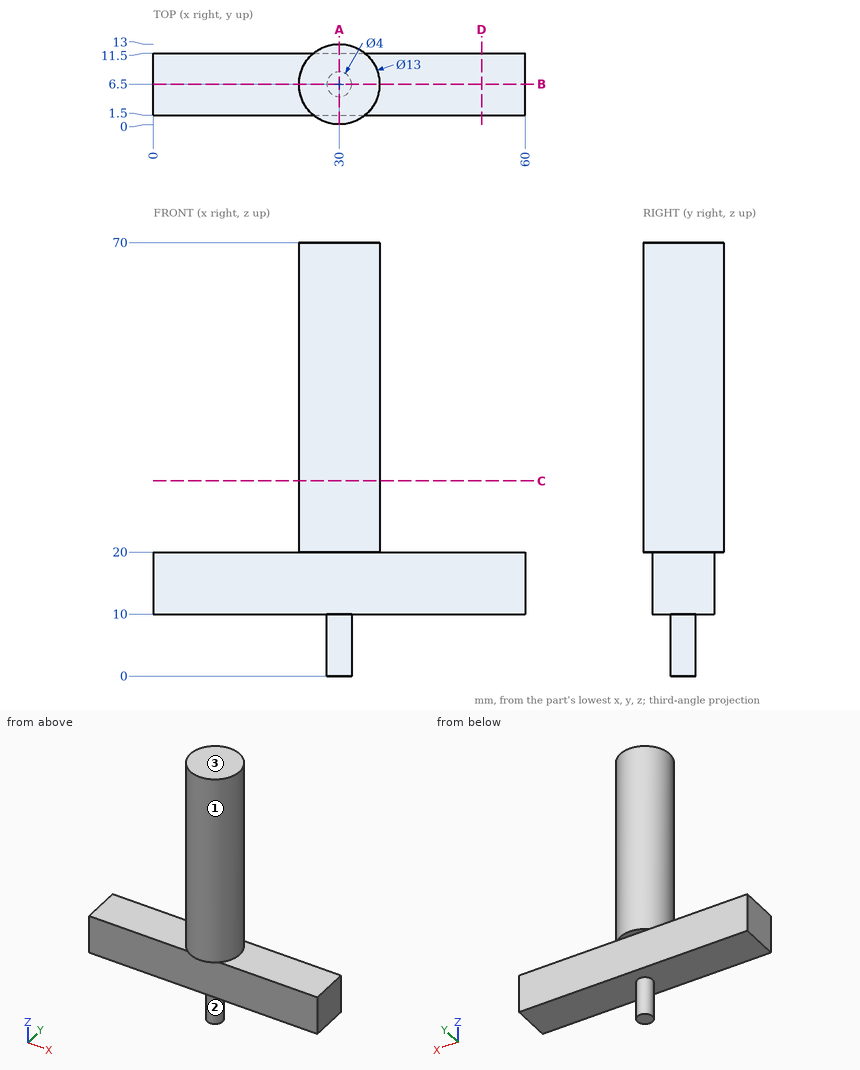
Geometry: see drawing. Coordinates: mm, zero at the bounding-box minimum. A direction names the side the tool comes from. Round coordinates to 2 decimals unless told otherwise and drop trailing zeros. Loops run counter-clockwise (first coordinate to the right, second up) from the corner with the lowest first, then second, coordinate; pieces in that order, holes last. Notation, with made-up numbers: M -21.75,53 L 3.25,53 A25 ccw 3.25,89 Z; hole C 10.5,35 d7. An arc over 180 degrees is marked long. Use a Markdown table: item, result. Add a question column.
1. Section query B-B on y = 6.5. Return the cut outline in (x, z), then the cut area to 3 significant figures.
2. Contact query for flat-ended pins moving along their axis: P1, Ø1.2, axis at x = 29, y = 12.5, coming from the -Z side; P2, Ø12, axis at x = 19.5, z = 43, coming from the +Y side; P3, Ø11, axis at x = 38.5, z = 13.5, coming from the -Y side. Output: stop coordinate, or through.
3. Section query A-A on x = 30. Return the cut outline in (y, z), then the cut area to 3 significant figures.
4. Line query: line 1 (Z direction, x = 45.5, y = 2.25); line 2 (Z direction, x = 34, y = 9); line 3 (X direction, y = 10.75, z = 33). Output: solid intervals per line, ascending.
5. Section query C-C on z = 31.5. Return the cut outline in (x, y), then the cut area to 3 significant figures.
6. Section query D-D on x = 53. Return the cut outline in (y, z).
7. Reachability of the marked faces 1, 2 and 3 from +Z, -Z, +X, -X, +Y, -Y: full face, straight path, thin tool, end or side. Return the list, or none.
Reported:
| question | item | result |
|---|---|---|
| 1 | outline | M 0,10 L 28,10 L 28,0 L 32,0 L 32,10 L 60,10 L 60,20 L 36.5,20 L 36.5,70 L 23.5,70 L 23.5,20 L 0,20 Z |
| 1 | area | 1,290 mm² |
| 2 | P1 | stops at z = 20 |
| 2 | P2 | stops at y = 11.19 |
| 2 | P3 | stops at y = 1.5 |
| 3 | outline | M 0,20 L 1.5,20 L 1.5,10 L 4.5,10 L 4.5,0 L 8.5,0 L 8.5,10 L 11.5,10 L 11.5,20 L 13,20 L 13,70 L 0,70 Z |
| 3 | area | 790 mm² |
| 4 | line 1 | z = 10 to 20 |
| 4 | line 2 | z = 10 to 70 |
| 4 | line 3 | x = 25.08 to 34.92 |
| 5 | outline | C 30,6.5 d13 |
| 5 | area | 133 mm² |
| 6 | outline | M 1.5,10 L 11.5,10 L 11.5,20 L 1.5,20 Z |
| 7 | face 1 | +Z |
| 7 | face 2 | -Z |
| 7 | face 3 | +Z, +X, -X, +Y, -Y |
